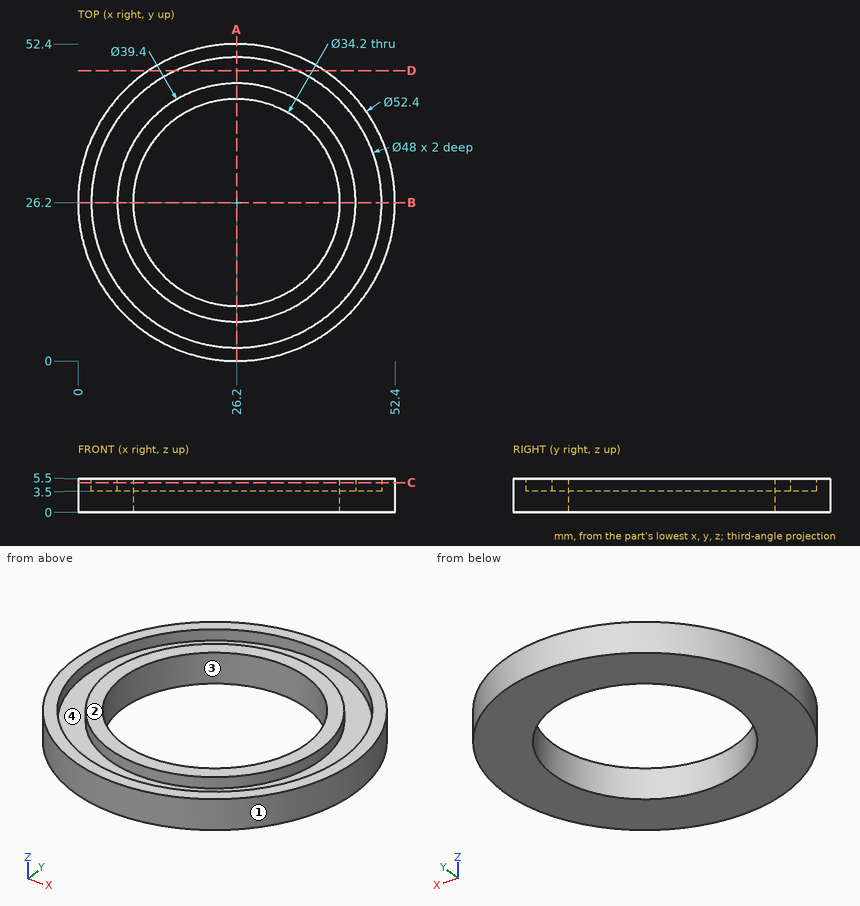
Print and shaded views of the part. All mm, measured from the part's lowest x, y and z. Give positions to 0.01 mm unless a question says otherwise; leave off trailing zeros. Loops run counter-clockwise (first coordinate to the right, second up) from the corner with the lowest first, then second, coordinate; pieces in that order, holes last.
1) Saw through at C-C (z = 4.9). Write the cut outline in (x, y).
2) Saw through at A-A (x = 26.2). Write the cut outline in (y, z).
3) Flat gauge pins, fed straight in: pin 1 Ø1 at (x, z) = (43, 1) entering from -Y; pin 2 Ø3 at (x, z) = (27, 5) entering from +Y. Where does each tip first touch, or does it go through?
4) Wall check: line 1 (Y direction, x = 26.2, z = 5); line 2 (X direction, y = 14, z = 4); line 3 (Y direction, x = 32.5, z = 4.9). Give the ranges that are in metal, low to high.
5) Saw through at D-D (y = 48). Write the cut outline in (x, z), plus the area to 3 significant figures.
6) Pull direction X, two halves, no side cores. Call the marked faces 1, 2, 3 and 4: +X half, -X half, draft (parallel to the pull), parting line (faces both ways), or undercut.
Answer block:
1. outline: circle Ø52.4 at (26.2, 26.2); circle Ø39.4 at (26.2, 26.2); hole circle Ø48 at (26.2, 26.2); hole circle Ø34.2 at (26.2, 26.2)
2. outline: (0, 0) - (9.1, 0) - (9.1, 5.5) - (6.5, 5.5) - (6.5, 3.5) - (2.2, 3.5) - (2.2, 5.5) - (0, 5.5) - close; (43.3, 0) - (52.4, 0) - (52.4, 5.5) - (50.2, 5.5) - (50.2, 3.5) - (45.9, 3.5) - (45.9, 5.5) - (43.3, 5.5) - close
3. pin 1: stops at y = 5.69
3. pin 2: stops at y = 52.4
4. line 1: y = 0 to 2.2, 6.5 to 9.1, 43.3 to 45.9, 50.2 to 52.4
4. line 2: x = 3.01 to 5.53, 10.73 to 14.22, 38.18 to 41.67, 46.87 to 49.39
4. line 3: y = 0.77 to 3.04, 7.53 to 10.3, 42.1 to 44.87, 49.36 to 51.63
5. outline: (11.67, 0) - (40.73, 0) - (40.73, 5.5) - (36.24, 5.5) - (36.24, 3.5) - (16.16, 3.5) - (16.16, 5.5) - (11.67, 5.5) - close
5. area: 120 mm2
6. face 1: parting line
6. face 2: draft
6. face 3: undercut
6. face 4: undercut
